from build123d import *

# Parameters (mm, degrees)
SKETCH1_R           = 2.032
SKETCH1_R_2         = 3.302
BOSS_EXTRUDE1_DEPTH = 2.54


with BuildPart() as part:
    # Sketch1 → Boss-Extrude1 (new body)
    with BuildSketch(Plane(origin=(0, 0, 0), x_dir=(1, 0, 0), z_dir=(0, 1, 0))):
        with BuildLine():
            Line((-20.290276596, 2.465366843), (-11.033687943, 11.413735382))
            ThreePointArc((-11.033687943, 11.413735382), (0, 15.875), (11.033687943, 11.413735382))
            Line((11.033687943, 11.413735382), (20.290276596, 2.465366843))
            ThreePointArc((20.290276596, 2.465366843), (21.336, 0), (20.290276596, -2.465366843))
            Line((20.290276596, -2.465366843), (11.033687943, -11.413735382))
            ThreePointArc((11.033687943, -11.413735382), (0, -15.875), (-11.033687943, -11.413735382))
            Line((-11.033687943, -11.413735382), (-20.290276596, -2.465366843))
            ThreePointArc((-20.290276596, -2.465366843), (-21.336, 0), (-20.290276596, 2.465366843))
        make_face()
        with Locations(Location((-17.907, 0, 0), (0, 0, 270))):
            Circle(SKETCH1_R, mode=Mode.SUBTRACT)
        with Locations(Location((17.907, 0, 0), (0, 0, 270))):
            Circle(SKETCH1_R, mode=Mode.SUBTRACT)
        with Locations(Location((0, 0, 0), (0, 0, 270))):
            Circle(SKETCH1_R_2, mode=Mode.SUBTRACT)
    extrude(amount=BOSS_EXTRUDE1_DEPTH)

    # Sketch3 → Revolve1 (revolve)
    with BuildSketch(Plane(origin=(0, 0, 0), x_dir=(0, 0, -1), z_dir=(1, 0, 0))):
        with BuildLine():
            Line((-3.302, 19.05), (-7.794998012, 19.05))
            add(Edge.make_bspline(
                [(-7.794998012, 19.05), (-10.740596789, 18.645101439), (-14.519445993, 10.395857778), (-5.018498512, 7.761963643), (-11.43, 2.54)],
                knots=[0, 0, 0, 0, 0.449937677, 1, 1, 1, 1], degree=3))
            Line((-11.43, 2.54), (-7.62, 2.54))
            Line((-7.62, 2.54), (-7.62, 12.7))
            Line((-7.62, 12.7), (-3.302, 12.7))
            Line((-3.302, 12.7), (-3.302, 19.05))
        make_face()
    revolve(axis=Axis((0, 19.05, 0), (0, -1, 0)))


solid = part.part
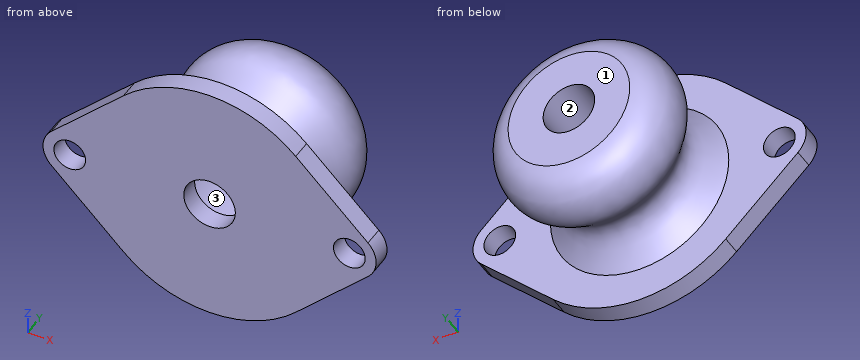
Read the model definition and answer for the solid it produces. Units are mm, in the model's axes. Face numbers are marked on the shaded views. Coordinates: 2 decimals unless noted, no trailing zeros. Order: outer loops, then holes, each group sorted by start corner. A loop starts at its lowest first (then second) coordinate and runs counter-clockwise, first axis right, second up. Notation, with made-up numbers: M 28.5,89.25 L 80.5,89.25 A17 cw 80.5,121.25 Z; hole C -17.75,-24 d11. An arc over 180 degrees is marked long. Put each result on its own line as item: value. Start each with the question number.
Item 1: Given pin 1 Ø2 at (y, z) = (11, 9.5) entering from -X; pin 2 Ø10 at (x, y) = (-1, 5.5) entering from -Z (3 decimals); pin 3 Ø10 at (y, z) = (8, 12) entering from -X; pin 4 Ø1 at (x, y) = (7, 11) entering from +Z, each flat-ended and moving along its own axis, determine where each tip first touches the part or whether it passes through.
Item 2: Consider probe 1 along Y at (x, z) = (5, 5.5); probe 2 along Z at (x, y) = (-5.5, 9); probe 3 along Y at (x, z) = (-1.5, -10.5). Determine where each line is inside the solid, lowest interval first. Write a range as [from, to].
Item 3: Section B-B, the plane x = -15 is taken. Determine the outline of the cut face in (y, z), plus the area to 3 significant figures.
Item 4: Section C-C, the plane x = 13.5 is taken. Determine the outline of the cut face in (y, z).
Item 5: Section A-A, the plane z = 0 is taken. Count the separate pieces of the cut face and the enclosed holes in it, plus the area to 3 significant figures.
Item 6: The mould has two halves that part along Y. Classify the marked faces 1, 2 and 3: +Y half, -Y half, draft (parallel to the pull), parting line (faces both ways), or undercut.
Computed:
1. pin 1: stops at x = -6.85
1. pin 2: stops at z = -15.875
1. pin 3: stops at x = -7.1
1. pin 4: stops at z = 8.66
2. probe 1: y = [0, 2.54], [12.7, 19.05]
2. probe 2: z = [-7.18, -5.27], [5.27, 7.18]
2. probe 3: y = [0, 3.25], [10.93, 17.31]
3. outline: M 0,-7.58 L 2.54,-7.58 L 2.54,7.58 L 0,7.58 Z
3. area: 38.5 mm2
4. outline: M 0,-9.03 L 2.54,-9.03 L 2.54,9.03 L 0,9.03 Z
5. separate pieces: 4
5. enclosed holes: 0
5. area: 209 mm2
6. face 1: +Y half
6. face 2: draft
6. face 3: undercut
